The model under review builds one solid part; all positions refer to its coordinate system, in mm. A direction names the side the tool comes from. Give positions to 0.01 mm unless a question says otherwise; leave off trailing zeros. Loops run counter-clockwise (first coordinate to the right, second up) from the corner with the lowest first, then second, coordinate; pieces in that order, holes last. Notation, with made-up numbers: M 28.25,-2.75 L 74.25,-2.75 A27 cw 74.25,17.25 Z; hole C -30,34.5 d1. An arc over 180 degrees is marked long. Return JSON: item names as keys, results as strings. Group by question number.
Autodesk Inventor part; units mm, degrees
ref_plane "YZ Plane" through (0, 0, 0) normal (1, 0, 0) x (0, 1, 0)
ref_plane "XZ Plane" through (0, 0, 0) normal (0, 1, 0) x (-1, 0, 0)
ref_plane "XY Plane" through (0, 0, 0) normal (0, 0, 1) x (1, 0, 0)
sketch "Plate" plane through (0, 0, 0) normal (0, 0, 1) x (1, 0, 0)
  line L0 (-200, -200) -> (200, -200) construction
  line L1 (200, -200) -> (200, 200) construction
  line L2 (200, 200) -> (-200, 200) construction
  line L3 (-200, 200) -> (-200, -200) construction
  line L4 (-200, -200) -> (200, 200) construction
  line L5 (200, -200) -> (-200, 200) construction
  line L6 (0, 0) -> (0, 420.657) construction
  line L7 (0, 0) -> (461.6465, 0) construction
  line L8 (0, 202) -> (202, 202) construction
  line L9 (202, 202) -> (202, 0) construction
  line L10 (74.8189, 0) -> (251.7605, 230.5948) construction
  line L11 (254.8388, 145.1612) -> (158.001, 241.999) construction
  line L12 (252.9755, 175.3088) -> (179.3809, 248.9034) construction
  line L13 (74.8189, 0) -> (228.2843, 200)
  line L14 (200, 200) -> (231.4665, 231.4665) construction
  line L15 (228.2843, 200) -> (214.1421, 214.1421)
  line L16 (200, 228.2843) -> (214.1421, 214.1421)
  line L17 (200, 228.2843) -> (0, 74.8189)
  line L18 (-74.8189, 0) -> (-228.2843, 200)
  line L19 (-228.2843, 200) -> (-214.1421, 214.1421)
  line L20 (-200, 228.2843) -> (-214.1421, 214.1421)
  line L21 (-200, 228.2843) -> (0, 74.8189)
  line L22 (74.8189, 0) -> (228.2843, -200)
  line L23 (228.2843, -200) -> (214.1421, -214.1421)
  line L24 (200, -228.2843) -> (214.1421, -214.1421)
  line L25 (200, -228.2843) -> (0, -74.8189)
  line L26 (-200, -228.2843) -> (0, -74.8189)
  line L27 (-200, -228.2843) -> (-214.1421, -214.1421)
  line L28 (-228.2843, -200) -> (-214.1421, -214.1421)
  line L29 (-74.8189, 0) -> (-228.2843, -200)
  dimension "d136" = 10
  dimension "d12" = 200
  dimension "d79" = 200
  dimension "d80" = 2
  dimension "d81" = 2
  dimension "d83" = 20
  dimension "d84" = 7.5
  dimension "d85" = 20
  dimension "d86" = 7.5
extrude "Base" add sketch "Plate" along normal blind 6.35
sketch "Sketch3" plane through (0, 0, 0) normal (0, 0, 1) x (1, 0, 0)
  line L0 (-70.7107, 0) -> (0, 70.7107)
  line L1 (0, 70.7107) -> (70.7107, 0)
  line L2 (70.7107, 0) -> (0, -70.7107)
  line L3 (0, -70.7107) -> (-70.7107, 0)
  line L4 (-70.7107, 0) -> (70.7107, 0) construction
  line L5 (0, 70.7107) -> (0, -70.7107) construction
  point P0 (0, 0)
  dimension "d76" = 90
  dimension "d77" = 100
extrude "Center hole" cut sketch "Sketch3" along normal through all
fillet "Fillet2" radius 75 4 edges at (0, 74.8189, 3.175) (-74.8189, 0, 3.175) (0, -74.8189, 3.175) (74.8189, 0, 3.175)
fillet "Fillet3" radius 35 4 edges at (-70.7107, 0, 3.175) (0, 70.7107, 3.175) (70.7107, 0, 3.175) (0, -70.7107, 3.175)
fillet "Fillet4" radius 10 8 edges at (200, 228.2843, 3.175) (228.2843, 200, 3.175) (228.2843, -200, 3.175) (200, -228.2843, 3.175) (-200, -228.2843, 3.175) (-228.2843, -200, 3.175) (-200, 228.2843, 3.175) (-228.2843, 200, 3.175)
sketch "Sketch17" plane through (0, 0, 0) normal (0, 0, 1) x (1, 0, 0)
  line L0 (-200, -200) -> (200, 200) construction
  line L1 (254.8388, 145.1612) -> (158.001, 241.999) construction
  line L2 (182.3223, 182.3223) -> (174.6892, 189.9555)
  line L3 (174.6892, 189.9555) -> (98.6702, 131.6241)
  line L4 (98.6702, 131.6241) -> (115.1472, 115.1472)
  line L5 (193.0425, 222.9456) -> (45.6571, 109.8528) construction
  line L6 (182.3223, 182.3223) -> (189.9555, 174.6892)
  line L7 (189.9555, 174.6892) -> (131.6241, 98.6702)
  line L8 (131.6241, 98.6702) -> (115.1472, 115.1472)
  point P0 (0, 0)
  dimension "d133" = 15
  dimension "d134" = 25
  dimension "d135" = 95
extrude "Extrusion4" cut sketch "Sketch17" along normal through all
fillet "Fillet5" radius 10 4 edges at (174.6892, 189.9555, 3.175) (189.9555, 174.6892, 3.175) (131.6241, 98.6702, 3.175) (98.6702, 131.6241, 3.175)
pattern_circular "Circular Pattern2" count 4 over 360 about axis through (0, 0, -10) along (0, 0, 1) of "Extrusion4", "Fillet5"
sketch "Sketch18" plane through (0, 0, 0) normal (0, 0, 1) x (1, 0, 0)
  arc A0 (-45.6571, 109.8528) -> (45.6571, 109.8528) centre (0, 169.3543) ccw construction
  line L0 (-20, 97.0701) -> (-20, 117.5)
  line L1 (-20, 117.5) -> (-55.6231, 117.5)
  line L2 (-69.5, 100.125) -> (-72.5, 100.125)
  arc A1 (-69.5, 92.875) -> (-69.5, 98.125) centre (-69.5, 95.5) ccw construction
  line L3 (-45.6571, 109.8528) -> (-193.0425, 222.9456) construction
  line L4 (-55.6231, 117.5) -> (-45.6571, 109.8528)
  arc A2 (-45.6571, 109.8528) -> (-20, 97.0701) centre (0, 169.3543) ccw
  point P0 (0, 0)
  dimension "d144" = 20
  dimension "d146" = 22
extrude "Limit nub" add sketch "Sketch18" along normal up to surface (6.35 mm away)
fillet "Fillet6" radius 5 3 edges at (-55.6231, 117.5, 3.175) (-20, 97.0701, 3.175) (-20, 117.5, 3.175)
properties part number "6061 Bed no holes" material "Aluminum 6061"
(1) Add section D-D (y = 152). Write out the cut boundary in (x, z).
(2) Add section A-A (y = -9). Write out the cut boundary in (x, z), and give its area (3 significant figures).
(3) Mouldability with a two-part tool opening along Y and no side actions: class faces 4 (the cylindrical face through (94.357, 0.687, 3.219)), 5 (the flat face through (-126, 171.5, 3.1)), 6 (the flat face through (-120.38, -167.19, 3.13)) as released by +Y, released by -Y, zero draft, split by the parting line, or undercut.
(4) For faces 1 (the flat face through (165.61, 118.32, 3.13)), 2 (the cylindrical face through (0.38, 56.21, 3.22)), 3 (the cylindrical face through (15.867, 96.052, 3.219)), list the 3-axis set-ups (+Z, -Z, +X, -X, +Y, -Y) from which the entire face can be reached by the end or side of a thin tool; tool diameter is ignored.
(5) Add section C-C (x = -174.5). Write out the cut boundary in (y, z).
(6) For probe 1 along Y at (x, z) = (-151, 2); probe 2 along X at (y, z) = (127.5, 1.25); probe 3 along Y at (x, z) = (122.5, 1), list the stretches that pass through material, from the lowest coordinate up.
(7) Add section B-B (x = 1). Write out the cut boundary in (y, z), and give its area (3 significant figures).
(8) For pin 1 (1.5 mm diameter, centred on y = 107.5, z = 4.5, fed in from +X); pin 2 (1 mm diameter, centred on x = -55.5, z = 1.5, fed in from +Y); pin 3 (1.9 mm diameter, centred on y = 106, z = 2.5, fed in from +X), all flat-tipped, find the tip position at first contact; note any pin that passes through.
Verdict:
{
 "1": {"outline": "M -191.45,0 L -172.55,0 L -172.55,6.35 L -191.45,6.35 Z; M -125.22,0 L -100.58,0 L -100.58,6.35 L -125.22,6.35 Z; M 100.58,0 L 125.22,0 L 125.22,6.35 L 100.58,6.35 Z; M 172.55,0 L 191.45,0 L 191.45,6.35 L 172.55,6.35 Z"},
 "2": {"outline": "M -94.9,0 L -55.04,0 L -55.04,6.35 L -94.9,6.35 Z; M 55.04,0 L 94.9,0 L 94.9,6.35 L 55.04,6.35 Z", "area": "506 mm²"},
 "3": {"face 4": "undercut", "face 5": "released by +Y", "face 6": "released by -Y"},
 "4": {"face 1": "+Z, -Z, +X", "face 2": "+Z, -Z", "face 3": "+Z, -Z, +Y"},
 "5": {"outline": "M -208.72,0 L -186.66,0 L -186.66,6.35 L -208.72,6.35 Z; M -154.55,0 L -129.91,0 L -129.91,6.35 L -154.55,6.35 Z; M 129.91,0 L 154.55,0 L 154.55,6.35 L 129.91,6.35 Z; M 186.66,0 L 208.72,0 L 208.72,6.35 L 186.66,6.35 Z"},
 "6": {"probe 1": "y = -190.69 to -171.78, -123.92 to -99.28, 99.28 to 123.92, 171.78 to 190.69", "probe 2": "x = -172.65 to -153.75, -104.31 to -68.66, 68.66 to 104.31, 153.75 to 172.65", "probe 3": "y = -168.82 to -149.91, -107.79 to -62.14, 62.14 to 107.79, 149.91 to 168.82"},
 "7": {"outline": "M -94.36,0 L -56.2,0 L -56.2,6.35 L -94.36,6.35 Z; M 56.2,0 L 94.36,0 L 94.36,6.35 L 56.2,6.35 Z", "area": "485 mm²"},
 "8": {"pin 1": "stops at x = 157.88", "pin 2": "stops at y = 117.95", "pin 3": "stops at x = 156.88"}
}
